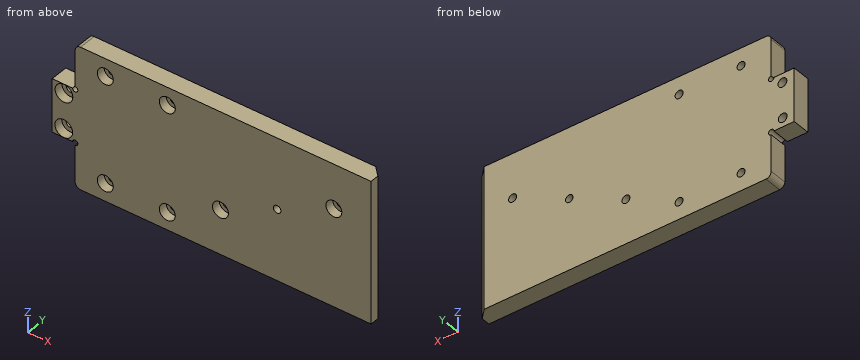
Solid Edge part; units mm, degrees
sketch "Sketch1" plane through (0, 0, 0) normal (0, -1, 0) x (1, 0, 0)
  line L0 (0, 0) -> (167, 0)
  line L1 (167, 0) -> (167, 80)
  line L2 (0, 80) -> (167, 80)
  line L3 (0, 55) -> (0, 80)
  line L4 (-13, 55) -> (0, 55)
  line L5 (-13, 25) -> (-13, 55)
  line L6 (0, 25) -> (-13, 25)
  line L7 (0, 0) -> (0, 25)
extrude "Protrusion1" add sketch "Sketch1" against normal blind 10
hole "Furo_1" at (0, 0, 55) direction (0, 1, 0) diameter 3 end up to next
hole "Hole1" at (0, 0, 25) direction (0, 1, 0) diameter 3 end up to next
hole "Furo_3" at (-6.4746, 0, 30.0331) direction (0, 1, 0) diameter 5 end up to next counterbore diameter 10 counterbore depth 5
hole "Hole2" at (-6.3505, 0, 49.8945) direction (0, 1, 0) diameter 5 end up to next counterbore diameter 10 counterbore depth 5
hole "Furo_7" at (17, 0, 70) direction (0, 1, 0) diameter 4.5 end up to next counterbore diameter 9 counterbore depth 5
hole "Hole3" at (52, 0, 70) direction (0, 1, 0) diameter 4.5 end up to next counterbore diameter 9 counterbore depth 5
hole "Hole4" at (52, 0, 9.8232) direction (0, 1, 0) diameter 4.5 end up to next counterbore diameter 9 counterbore depth 5
hole "Hole5" at (17, 0, 10) direction (0, 1, 0) diameter 4.5 end up to next counterbore diameter 9 counterbore depth 5
hole "Hole6" at (82, 0, 25) direction (0, 1, 0) diameter 4.5 end up to next counterbore diameter 9 counterbore depth 5
hole "Hole7" at (146, 0, 55) direction (0, 1, 0) diameter 4.5 end up to next counterbore diameter 9 counterbore depth 5
hole "Furo_13" at (114, 0, 40) direction (0, 1, 0) diameter 4.2 end through all
sketch "Sketch2" plane through (83.5, 5, 0) normal (0, 0, -1) x (1, 0, 0)
  line L0 (78.5, -5) -> (83.5, 0)
  line L1 (83.5, -5) -> (78.5, -5)
extrude "Recorte_Extrudado_1" cut sketch "Sketch2" against normal blind 110.0031 material side at (164.5354, 7.5354, 0)
fillet "Redondo_1" radius 3 2 edges at (0, 5, 0) (0, 5, 80)
properties material "PVC"
Geometry check sheet. Reference: the model listing, model coordinates, mm. Give positions to 0.01 mm unless a question says otherwise; leave off trailing zeros. Order: outer loops, then holes, each group sorted by start corner. A loop starts at its lowest first (then second) coordinate and runs counter-clockwise, first axis right, second up.
1) Cross-section at B-B (x = 146). Record the boundary of the cut face in (y, z), then the cut area to 4 significant figures.
Results are:
outline: (0, 0) - (10, 0) - (10, 52.75) - (5, 52.75) - (5, 50.5) - (0, 50.5) - close; (0, 59.5) - (5, 59.5) - (5, 57.25) - (10, 57.25) - (10, 80) - (0, 80) - close
area: 732.5 mm2
2) Gauge pin test, flat ends, axial feed: pin 1 (7 mm diameter, centred on x = 17.5, z = 70, fed in from -Y); pin 2 (3 mm diameter, centred on x = -5.5, y = 6, fed in from +Z); pin 3 (1 mm diameter, centred on y = 6.5, z = 56.5, fed in from +X); pin 4 (14.5 mm diameter, centred on x = 82, z = 25, fed in from +Y). Record the tip position at first contact, or that the pin passes through.
Results are:
pin 1: stops at y = 5
pin 2: stops at z = 55
pin 3: stops at x = 166
pin 4: stops at y = 10
3) Cross-section at A-A (z = 40). Record the boundary of the cut face in (x, y).
Results are:
outline: (-13, 0) - (111.9, 0) - (111.9, 10) - (-13, 10) - close; (116.1, 0) - (167, 0) - (167, 5) - (162, 10) - (116.1, 10) - close
4) Material ranges on probe 1 along X at (y, z) = (2.7, 70); probe 2 along Z at (x, y) = (52, 8.75); probe 3 along Z at (x, y) = (52, 2.35), recorded low to high.
Results are:
probe 1: x = 0 to 12.5, 21.5 to 47.5, 56.5 to 167
probe 2: z = 0 to 7.57, 12.07 to 67.75, 72.25 to 80
probe 3: z = 0 to 5.32, 14.32 to 65.5, 74.5 to 80
5) Cross-section at D-D (z = 10). Record the boundary of the cut face in (x, y).
Results are:
outline: (0, 0) - (12.5, 0) - (12.5, 5) - (14.75, 5) - (14.75, 10) - (0, 10) - close; (19.25, 5) - (21.5, 5) - (21.5, 0) - (47.5, 0) - (47.5, 5) - (49.76, 5) - (49.76, 10) - (19.25, 10) - close; (54.24, 5) - (56.5, 5) - (56.5, 0) - (167, 0) - (167, 5) - (162, 10) - (54.24, 10) - close
6) Cross-section at C-C (x = 17). Record the boundary of the cut face in (y, z).
Results are:
outline: (0, 0) - (10, 0) - (10, 7.75) - (5, 7.75) - (5, 5.5) - (0, 5.5) - close; (0, 14.5) - (5, 14.5) - (5, 12.25) - (10, 12.25) - (10, 67.75) - (5, 67.75) - (5, 65.5) - (0, 65.5) - close; (0, 74.5) - (5, 74.5) - (5, 72.25) - (10, 72.25) - (10, 80) - (0, 80) - close
